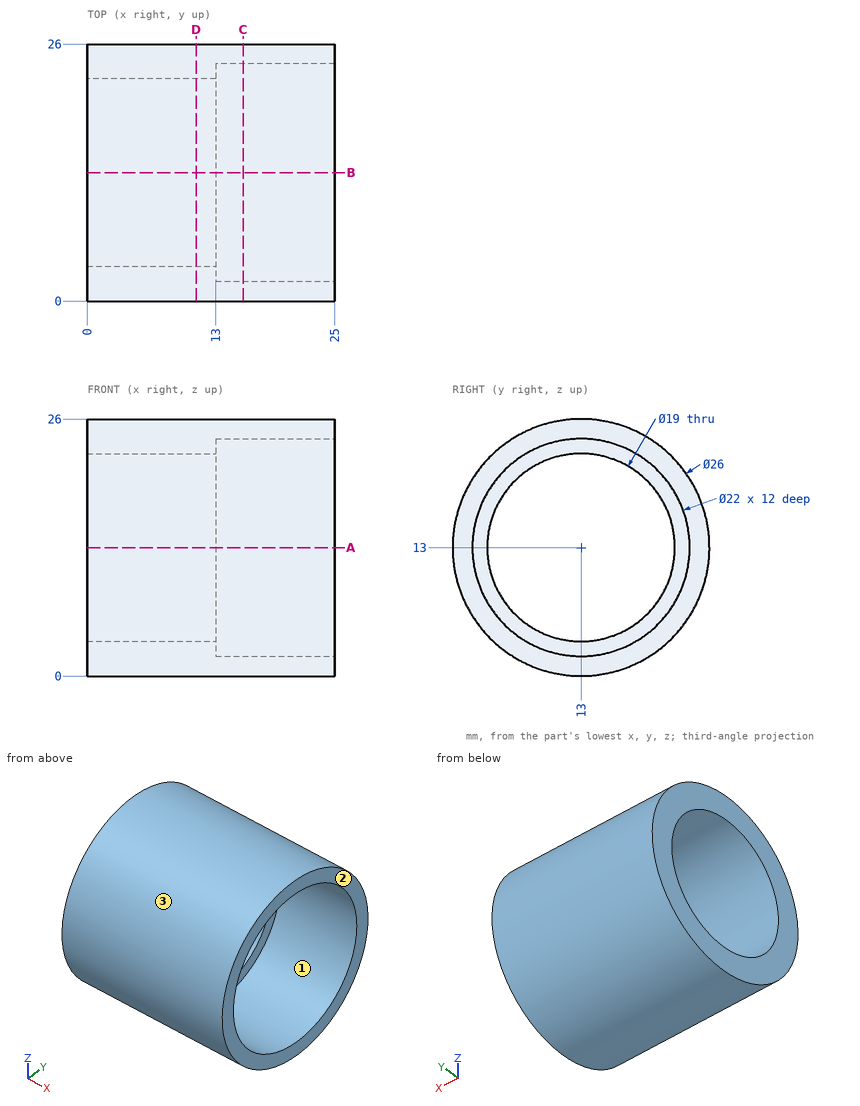
Can you work these out from the drawing? Everything is in mm from the part's minimum corner. Round coordinates to 2 decimals unless told otherwise and drop trailing zeros. Order: outer loops, then holes, each group sorted by start corner. A loop starts at its lowest first (then second) coordinate and runs counter-clockwise, first axis right, second up. Notation, with made-up numbers: (-35, -25.75) -> (-25, -25.75) arc R15 ccw to (-25, -0.75) -> close; hole circle Ø5 at (-12, -3.5). An arc over 180 degrees is marked (long way). Return JSON: item names as keys, results as strings. Group by question number.
1. If we section it at D-D, the plane x = 11: Write out the boundary of the cut face in (y, z).
2. We'd pull the mould along Y, two halves only. Please class the marked faces 1, 2 and 3: released by +Y, released by -Y, zero draft, split by the parting line, or undercut.
3. Will these pins go through, and if not, where does the flat tip stop? pin 1 (10 mm diameter, centred on y = 20.5, z = 8, fed in from +X); pin 2 (6 mm diameter, centred on x = 16, y = 21, fed in from -Z); pin 3 (8 mm diameter, centred on x = 11.5, y = 20, fed in from +Z); pin 4 (8 mm diameter, centred on x = 14.5, z = 19.5, fed in from -Y).
4. If we section it at C-C, the plane x = 15.75: Write out the boundary of the cut face in (y, z), then the cut area to 3 significant figures.
5. I need wall thicknesses on line 1 (Z direction, x = 4.5, y = 13); line 2 (Z direction, x = 21, y = 13). Which ranges of each line are inside material? Lowest first, please. Write a range as [from, to].
6. If we section it at A-A, the plane z = 13: Write out the boundary of the cut face in (x, y), then the cut area to 3 significant figures.
Output values:
{
 "1": {"outline": "circle Ø26 at (13, 13); hole circle Ø19 at (13, 13)"},
 "2": {"face 1": "undercut", "face 2": "zero draft", "face 3": "split by the parting line"},
 "3": {"pin 1": "x = 25", "pin 2": "z = 1", "pin 3": "z = 25.65", "pin 4": "y = 0.24"},
 "4": {"outline": "circle Ø26 at (13, 13); hole circle Ø22 at (13, 13)", "area": "151 mm²"},
 "5": {"line 1": "[0, 3.5], [22.5, 26]", "line 2": "[0, 2], [24, 26]"},
 "6": {"outline": "(0, 0) -> (25, 0) -> (25, 2) -> (13, 2) -> (13, 3.5) -> (0, 3.5) -> close; (0, 22.5) -> (13, 22.5) -> (13, 24) -> (25, 24) -> (25, 26) -> (0, 26) -> close", "area": "139 mm²"}
}
